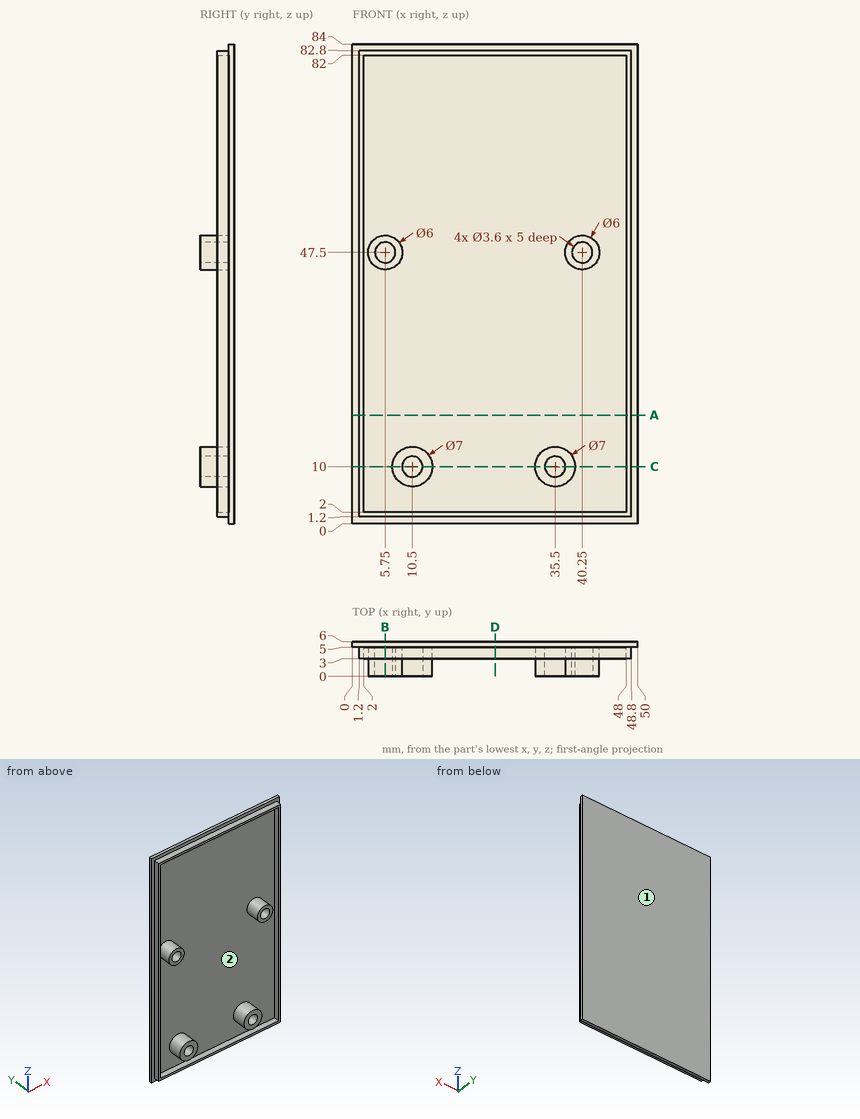
Input: dimensioned drawing with shaded views. Units: mm. Origin: part minimum x, y, z. Give positions to 0.01 mm unless a question says otherwise; leave off trailing zeros. Write each loop counter-clockwise with the first axis right and the second up, starting at its lowest first coordinate (ties: lowest second). Pieces come first, ordered by that corner, then holes. Notation, with made-up numbers: M 49,-12 L 72,-12 A25 cw 72,12 Z; hole C 1,50 d5. An arc over 180 degrees is marked long. Return JSON: item names as keys, results as strings. Group by question number.
1) Cut plane A-A, the plane z = 19. Output: boundary loops of the cut face in (x, y).
2) Material intervals for line 1 along Z through (x, y) = (5.75, 3.8); line 2 along Z through (x, y) = (10.5, 3.8); line 3 along X through (y, z) = (4.9, 72.5), sorted ascending. Write a range as [from, to].
3) Pull-direction query (Z, two-part tool) for the marked faces 1 and 2; classes: pulls with the +Z half, pulls with the -Z half, needs draft (parallel to the pull), parting line crosses it, or undercut.
4) Cut plane D-D, the plane x = 25. Output: boundary loops of the cut face in (y, z), plus the area to 3 significant figures.
5) Cut plane C-C, the plane z = 10. Output: boundary loops of the cut face in (x, y), plus the area to 3 significant figures.
6) Pin query (flat end, axial travel): P1, Ø1, axis at y = 3, z = 50, coming from the -X side; P2, Ø1.6, axis at x = 19.5, y = 3.5, coming from the -Z side; P3, Ø6, axis at x = 23, z = 29, coming from the -Y side. Return the tip coordinate at first contact, or that it passes through.
7) Cut plane B-B, the plane x = 5.75. Output: boundary loops of the cut face in (y, z), plus the area to 3 significant figures.
Recorded:
{
 "1": {"outline": "M 0,5 L 1.2,5 L 1.2,3 L 2,3 L 2,5 L 48,5 L 48,3 L 48.8,3 L 48.8,5 L 50,5 L 50,6 L 0,6 Z"},
 "2": {"line 1": "z = [1.2, 2], [44.5, 45.7], [49.3, 50.5], [82, 82.8]", "line 2": "z = [1.2, 2], [6.5, 8.2], [11.8, 13.5], [82, 82.8]", "line 3": "x = [1.2, 2], [48, 48.8]"},
 "3": {"face 1": "needs draft", "face 2": "undercut"},
 "4": {"outline": "M 3,1.2 L 5,1.2 L 5,0 L 6,0 L 6,84 L 5,84 L 5,82.8 L 3,82.8 L 3,82 L 5,82 L 5,2 L 3,2 Z", "area": "87.2 mm²"},
 "5": {"outline": "M 0,5 L 1.2,5 L 1.2,3 L 2,3 L 2,5 L 7,5 L 7,0 L 8.7,0 L 8.7,5 L 12.3,5 L 12.3,0 L 14,0 L 14,5 L 32,5 L 32,0 L 33.7,0 L 33.7,5 L 37.3,5 L 37.3,0 L 39,0 L 39,5 L 48,5 L 48,3 L 48.8,3 L 48.8,5 L 50,5 L 50,6 L 0,6 Z", "area": "87.2 mm²"},
 "6": {"P1": "stops at x = 1.2", "P2": "stops at z = 1.2", "P3": "stops at y = 5"},
 "7": {"outline": "M 0,44.5 L 5,44.5 L 5,2 L 3,2 L 3,1.2 L 5,1.2 L 5,0 L 6,0 L 6,84 L 5,84 L 5,82.8 L 3,82.8 L 3,82 L 5,82 L 5,50.5 L 0,50.5 L 0,49.3 L 5,49.3 L 5,45.7 L 0,45.7 Z", "area": "99.2 mm²"}
}
